from build123d import *

# Parameters (mm, degrees)
SKETCH1_W           = 12.065
SKETCH1_H           = 25.4762
BOSS_EXTRUDE1_DEPTH = 10.033
SKETCH2_R           = 1.49225
BOSS_EXTRUDE2_DEPTH = 10.033
CUT_EXTRUDE1_DEPTH  = 8.6106


with BuildPart() as part:
    # Sketch1 → Boss-Extrude1 (new body)
    with BuildSketch(Plane.XY):
        with Locations((6.0325, 12.7381)):
            Rectangle(SKETCH1_W, SKETCH1_H)
    extrude(amount=BOSS_EXTRUDE1_DEPTH)

    # Sketch2 → Boss-Extrude2 (add)
    with BuildSketch(Plane(origin=(0, 25.4762, 0), x_dir=(1, 0, 0), z_dir=(0, 1, 0))):
        with Locations((6.0325, -5.0165)):
            Circle(SKETCH2_R)
    extrude(amount=BOSS_EXTRUDE2_DEPTH)

    # Sketch3 → Cut-Extrude1 (cut)
    with BuildSketch(Plane(origin=(0, 35.5092, 0), x_dir=(1, 0, 0), z_dir=(0, 1, 0))):
        with BuildLine():
            Line((4.890142942, -4.05638), (7.174857058, -4.05638))
            ThreePointArc((7.174857058, -4.05638), (6.0325, -3.52425), (4.890142942, -4.05638))
        make_face()
    extrude(amount=-CUT_EXTRUDE1_DEPTH, mode=Mode.SUBTRACT)


solid = part.part
CAD build for the part. Positions are in the model's coordinates, mm. A direction names the side the tool comes from. Round coordinates to 2 decimals unless told otherwise and drop trailing zeros. Order: outer loops, then holes, each group sorted by start corner. A loop starts at its lowest first (then second) coordinate and runs counter-clockwise, first axis right, second up. Notation, with made-up numbers: (-37, -33) -> (-18, -33) arc R11 cw to (-18, -18) -> close; hole circle Ø9 at (32, 69). An arc over 180 degrees is marked (long way). Write item = value, one per line. Start each with the question number.
(1) Cut at C-C, the plane x = 3.5. List the corners of the cut face in (y, z).
(2) Pin check, flat tips, straight feed: P1, Ø3, axis at x = 10, z = 6, coming from the +Y side; P2, Ø1.1, axis at x = 5.5, y = 32, coming from the -Z side; P3, Ø3, axis at y = 29.5, z = 7.5, coming from the +X side; P4, Ø1, axis at x = 9.5, y = 29, coming from the -Z side. Stop position of each tip, or through.
(3) Cut at B-B, the plane z = 8.5. List the corners of the cut face in (x, y) (3 decimals), then the cut area to 3 significant figures.
(4) Probe line 1 (Y direction, x = 8.5, z = 8). List the from-to ranges inside material, lowest first. Write a range as [from, to].
(5) Cut at A-A, the plane y = 30.5. List the corners of the cut face in (x, z).
(6) Cut at D-D, the plane y = 26. List the corners of the cut face in (x, z).
(7) Which spindle directions (+Z, -Z, +X, -X, +Y, -Y) get a long thin tool onto all of the face, cutting with end or side? Do faces 1 (the flat face through (6, 13, 0)), 2 (the flat face through (4.6, 25.476, 3.8)), 3 (the flat face through (6, 31, 4.056)). Say none if no direction does.
Model answer:
q1.outline = (0, 0) -> (25.48, 0) -> (25.48, 10.03) -> (0, 10.03) -> close
q2.P1 = 25.48
q2.P2 = 4.06
q2.P3 = 7.15
q2.P4 = through
q3.outline = (0, 0) -> (12.065, 0) -> (12.065, 25.476) -> (0, 25.476) -> close
q3.area = 307 mm2
q4.line_1 = [0, 25.48]
q5.outline = (4.89, 4.06) -> (7.17, 4.06) arc R1.49 ccw (long way) to start
q6.outline = circle Ø2.98 at (6.03, 5.02)
q7.face_1 = -Z, +X, -X, +Y, -Y
q7.face_2 = +Y
q7.face_3 = -Z, +X, -X, +Y
